from build123d import *

# Parameters (mm, degrees)
SKETCH_1_W      = 120
SKETCH_1_H      = 60
EXTRUDE_1_DEPTH = 7.6
SKETCH_5_W      = 130
SKETCH_5_H      = 60
EXTRUDE_2_DEPTH = 1.6
FILLET_1_R      = 2


with BuildPart() as part:
    # 草图1 → 凸台-拉伸1 (new body)
    with BuildSketch(Plane.XY):
        Rectangle(SKETCH_1_W, SKETCH_1_H)
    extrude(amount=EXTRUDE_1_DEPTH)

    # 草图5 → 凸台-拉伸2 (add)
    with BuildSketch(Plane(origin=(0, 0, 0), x_dir=(-1, 0, 0), z_dir=(0, 0, -1))):
        Rectangle(SKETCH_5_W, SKETCH_5_H)
    extrude(amount=-EXTRUDE_2_DEPTH)

    # 圆角1
    fillet_1_edges = [part.edges().sort_by_distance(p)[0] for p in [
        (65, 30, 0.8),
        (-65, -30, 0.8),
        (65, -30, 0.8),
        (-65, 30, 0.8),
    ]]
    fillet(fillet_1_edges, radius=FILLET_1_R)


solid = part.part
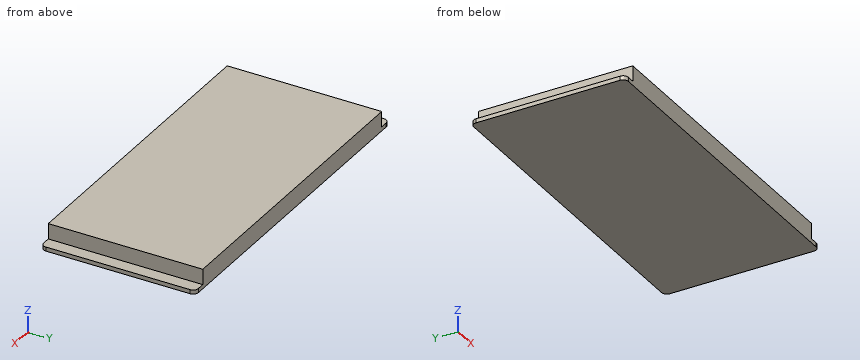
Source: CAD feature listing. Evaluate the final solid. Frame: model axes, mm. Give positions to 0.01 mm unless a question says otherwise; leave off trailing zeros. Order: outer loops, then holes, each group sorted by start corner. A loop starts at its lowest first (then second) coordinate and runs counter-clockwise, first axis right, second up. Notation, with made-up numbers: (45.25, 31) -> (62.25, 31) arc R30 ccw to (62.25, 58) -> close; hole circle Ø3 at (-33, -28.75). An arc over 180 degrees is marked (long way). Write item = value, one per line.
Item 1: Contact query for flat-ended pins moving along their axis: pin 1 (1 mm diameter, centred on y = -13.5, z = 5.5, fed in from -X); pin 2 (4 mm diameter, centred on x = 45, y = 20.5, fed in from -Z); pin 3 (1.8 mm diameter, centred on y = -8.5, z = 5.5, fed in from +X). Output: stop coordinate, or through.
Check result:
pin_1 = -60
pin_2 = 0
pin_3 = 60
Item 2: Section query B-B (z = 6.25). Output: boundary loops of the cut face in (x, y).
Check result:
outline = (-60, -30) -> (60, -30) -> (60, 30) -> (-60, 30) -> close
Item 3: Ray query, probe 1 along X at (y, z) = (20, 3). Return the intervals inside material, ascending.
Check result:
probe_1 = -60 to 60
Item 4: Section query A-A (y = 1.5). Output: boundary loops of the cut face in (x, z).
Check result:
outline = (-65, 0) -> (65, 0) -> (65, 1.6) -> (60, 1.6) -> (60, 7.6) -> (-60, 7.6) -> (-60, 1.6) -> (-65, 1.6) -> close
